```python
from build123d import *

# Parameters (mm, degrees)
BOSS_EXTRUDE1_DEPTH               = 18.2
SKETCH1_3_W                       = 18.5
SKETCH1_3_H                       = 70.5
SKETCH1_3_W_2                     = 3
SKETCH1_3_H_2                     = 2.475
BOSS_EXTRUDE2_DEPTH               = 5.5
FILLET1_R                         = 9
SKETCH4_W                         = 11.75
SKETCH4_H                         = 3
CUT_EXTRUDE1_DEPTH                = 103
TAP_DRILL_FOR_M3_TAP1_D           = 2.5
TAP_DRILL_FOR_M3_TAP1_CSINK_D     = 2.55
TAP_DRILL_FOR_M3_TAP1_CSINK_ANGLE = 90
FILLET2_R                         = 9


with BuildPart() as part:
    # Sketch1 → Boss-Extrude1 (new body)
    with BuildSketch(Plane.XY):
        Polygon((1.5, -37.725), (22.5, -37.725), (22.5, 37.725), (-22.5, 37.725), (-22.5, -37.725), (-1.5, -37.725), (-1.5, -35.25), (-9.25, -35.25), (-9.25, 35.25), (9.25, 35.25), (9.25, -35.25), (1.5, -35.25), align=None)
    extrude(amount=BOSS_EXTRUDE1_DEPTH)

    # Sketch1_3 → Boss-Extrude2 (add)
    with BuildSketch(Plane.XY):
        Polygon((1.5, -37.725), (22.5, -37.725), (22.5, 37.725), (-22.5, 37.725), (-22.5, -37.725), (-1.5, -37.725), (-1.5, -35.25), (-9.25, -35.25), (-9.25, 35.25), (9.25, 35.25), (9.25, -35.25), (1.5, -35.25), align=None)
        Rectangle(SKETCH1_3_W, SKETCH1_3_H)
        with Locations((0, -36.4875)):
            Rectangle(SKETCH1_3_W_2, SKETCH1_3_H_2)
    extrude(amount=-BOSS_EXTRUDE2_DEPTH)

    # Fillet1
    fillet1_edges = [part.edges().sort_by_distance(p)[0] for p in [
        (-9.25, 0, 0),
        (9.25, 0, 0),
    ]]
    fillet(fillet1_edges, radius=FILLET1_R)

    # Sketch4 → Cut-Extrude1 (cut)
    with BuildSketch(Plane.XZ.offset(37.725)):
        with Locations((5.875, -4)):
            Rectangle(SKETCH4_W, SKETCH4_H)
        Polygon((11.75, 15.7), (11.75, -2.5), (11.75, -5.5), (22.5, -5.5), (22.5, 15.7), align=None)
        with Locations((-5.875, -4)):
            Rectangle(SKETCH4_W, SKETCH4_H)
        Polygon((-11.75, 15.7), (-22.5, 15.7), (-22.5, -5.5), (-11.75, -5.5), (-11.75, -2.5), align=None)
    extrude(amount=-CUT_EXTRUDE1_DEPTH, mode=Mode.SUBTRACT)

    # Tap Drill for M3 Tap1 (through all)
    with Locations(Plane(origin=(0, 0, -5.5), x_dir=(-1, 0, 0), z_dir=(0, 0, -1))):
        with Locations((19.999953282, 35.25), (-20.000046718, 35.25), (-20.000046718, -29.75), (19.999953282, -29.75)):
            CounterSinkHole(TAP_DRILL_FOR_M3_TAP1_D / 2, TAP_DRILL_FOR_M3_TAP1_CSINK_D / 2, counter_sink_angle=TAP_DRILL_FOR_M3_TAP1_CSINK_ANGLE)

    # Fillet2
    fillet2_edges = [part.edges().sort_by_distance(p)[0] for p in [
        (-11.75, 0, -2.5),
        (11.75, 0, -2.5),
    ]]
    fillet(fillet2_edges, radius=FILLET2_R)


solid = part.part
```
Geometry check sheet. Reference: the model listing, model coordinates, mm. A direction names the side the tool comes from. Coordinates: 2 decimals unless noted, no trailing zeros. Order: outer loops, then holes, each group sorted by start corner. A loop starts at its lowest first (then second) coordinate and runs counter-clockwise, first axis right, second up. Notation, with made-up numbers: (37, 87) - (79, 87) arc R12 ccw to (79, 105) - close; hole circle Ø4 at (16.5, -23.5). An arc over 180 degrees is marked (long way). Answer as a JSON object with one key per item and string values. Group by question number.
Item 1: Tool access check on faces 4 (the face through (17, -1, 15.7)), 5 (the face through (-11.75, -1, 11)), 6 (the face through (1.5, -36, 9)), 7 (the face through (9.25, 0, 14)). Record the directions out of +Z, -Z, +X, -X, +Y, -Y that give a thin tool (end or side, any length) a straight path to the whole face; none if there is none.
Item 2: Sectioned sample at A-A, the plane y = -29.75. Record the cut outline in (x, z).
Item 3: Draft check along X on faces 1 (the face through (-22.5, 1, 17)), 2 (the face through (0, 37.725, 10)), 3 (the face through (-19, -29, 17)). Enter one of: +X half, -X half, draft (parallel to the pull), parting line (faces both ways), or undercut.
Item 4: Sectioned sample at B-B, the plane x = 19.5. Record the cut outline in (y, z) (3 decimals), and give its area (3 significant figures).
Item 5: Scan lines: probe 1 along X at (y, z) = (3, 9); probe 2 along Y at (x, z) = (-2.5, 2) (3 decimals). Record each from-to range of solid material in increasing order.
Item 6: Sectioned sample at C-C, the plane y = 30.5. Record the cut outline in (x, z).
Item 7: Sectioned sample at D-D, the plane z = 3.5. Record the cut outline in (x, y) (3 decimals).
Item 8: Depth check by flat-ended pin: pin 1 Ø3 at (x, y) = (18.5, 10) entering from -Z; pin 2 Ø0.7 at (y, z) = (-36.5, 10) entering from -X; pin 3 Ø8 at (y, z) = (26.5, 2) entering from +X. Enter the tip coordinate at first touch or a pass-through.
Resolved:
{
 "1": {"face 4": "-Z, +X, +Y, -Y", "face 5": "-Z, -X, +Y, -Y", "face 6": "+Z, -Y", "face 7": "+Z"},
 "2": {"outline": "(-22.5, 15.7) - (-21.25, 15.7) - (-21.25, 18.2) - (-22.5, 18.2) - close; (-18.75, 15.7) - (-11.75, 15.7) - (-11.75, 6.5) arc R9 ccw to (-2.75, -2.5) - (2.75, -2.5) arc R9 ccw to (11.75, 6.5) - (11.75, 15.7) - (18.75, 15.7) - (18.75, 18.2) - (9.25, 18.2) - (9.25, 9) arc R9 cw to (0.25, 0) - (-0.25, 0) arc R9 cw to (-9.25, 9) - (-9.25, 18.2) - (-18.75, 18.2) - close; (21.25, 15.7) - (22.5, 15.7) - (22.5, 18.2) - (21.25, 18.2) - close"},
 "3": {"face 1": "-X half", "face 2": "draft", "face 3": "undercut"},
 "4": {"outline": "(-37.725, 15.7) - (-30.896, 15.7) - (-30.896, 18.2) - (-37.725, 18.2) - close; (-28.604, 15.7) - (34.104, 15.7) - (34.104, 18.2) - (-28.604, 18.2) - close; (36.396, 15.7) - (37.725, 15.7) - (37.725, 18.2) - (36.396, 18.2) - close", "area": "177 mm^2"},
 "5": {"probe 1": "-11.75 to -9.25, 9.25 to 11.75", "probe 2": "-37.725 to -35.25, 35.25 to 37.725"},
 "6": {"outline": "(-22.5, 15.7) - (-11.75, 15.7) - (-11.75, 6.5) arc R9 ccw to (-2.75, -2.5) - (2.75, -2.5) arc R9 ccw to (11.75, 6.5) - (11.75, 15.7) - (22.5, 15.7) - (22.5, 18.2) - (9.25, 18.2) - (9.25, 9) arc R9 cw to (0.25, 0) - (-0.25, 0) arc R9 cw to (-9.25, 9) - (-9.25, 18.2) - (-22.5, 18.2) - close"},
 "7": {"outline": "(-11.235, -37.725) - (-1.5, -37.725) - (-1.5, -35.25) - (-7.374, -35.25) - (-7.374, 35.25) - (7.374, 35.25) - (7.374, -35.25) - (1.5, -35.25) - (1.5, -37.725) - (11.235, -37.725) - (11.235, 37.725) - (-11.235, 37.725) - close"},
 "8": {"pin 1": "z = 15.7", "pin 2": "x = -11.75", "pin 3": "x = 11.74"}
}
